Geometry check sheet. Reference: the model listing, model coordinates, mm. A direction names the side the tool comes from. Give positions to 0.01 mm unless a question says otherwise; leave off trailing zeros. Loops run counter-clockwise (first coordinate to the right, second up) from the corner with the lowest first, then second, coordinate; pieces in that order, holes last. Notation, with made-up numbers: (37, 67) -> (67, 67) arc R16 ccw to (67, 85) -> close; hole circle Ø5 at (32, 30.5). An arc over 180 degrees is marked (long way). Write each question's results on one line, items separated by ' | '. Start each with the question number.
1) Draft check along Z on faces 1 (the face through (0, 2, 1)), 2 (the face through (-1, -5.5, 2)), 3 (the face through (0, 0, 4)). Enter one of: pulls with the +Z half, pulls with the -Z half, needs draft (parallel to the pull), parting line crosses it, or undercut.
2) Scan lines: line 1 (Z direction, x = 0, y = -0.75); line 2 (Z direction, x = 0, y = 4.25). Record each from-to range of solid material in increasing order. Write a range as from..to.
3) Sectioned sample at B-B on y = 0. Record the cut outline in (x, z), then the cut area to 3 significant figures.
4) Set-up check for faces 4 (the face through (2, 1.5, -2)), 5 (the face through (2, -1.5, -2)), 6 (the face through (-3.448, 0.021, -2.028)): record each of +Z, -Z, +X, -X, +Y, -Y from which the full face is reachable in a straight line by a thin tool's end or side.
5) Sectioned sample at A-A on x = 0. Record the cut outline in (y, z).
6) Sectioned sample at D-D on z = -3. Record the cut outline in (x, y).
7) Depth check by flat-ended pin: pin 1 (1 mm diameter, centred on x = -3.5, z = -1.5, fed in from +Y); pin 2 (4 mm diameter, centred on x = 2, y = 8, fed in from +Z); pin 3 (1 mm diameter, centred on y = -2.5, z = 0, fed in from -X). Enter the tip coordinate at first touch or a pass-through.
8) Sectioned sample at C-C on x = 3.75. Record the cut outline in (y, z), then the cut area to 3 significant figures.
```python
from build123d import *

# Parameters (mm, degrees)
BOSS_EXTRUDE1_DEPTH = 1.5
SKETCH4_R           = 2.5
BOSS_EXTRUDE3_DEPTH = 4
SKETCH2_R           = 2.5
BOSS_EXTRUDE2_DEPTH = 8
SKETCH3_R           = 1
CUT_EXTRUDE1_DEPTH  = 16
CHAMFER2_SIZE       = 1


with BuildPart() as part:
    # Sketch1 → Boss-Extrude1 (new body, symmetric)
    with BuildSketch(Plane(origin=(0, 0, 0), x_dir=(1, 0, 0), z_dir=(0, 1, 0))):
        Polygon((2.309401077, 4), (-2.309401077, 4), (-4.618802154, 0), (-2.309401077, -4), (2.309401077, -4), (4.618802154, 0), align=None)
    extrude(amount=BOSS_EXTRUDE1_DEPTH, both=True)

    # Sketch4 → Boss-Extrude3 (add)
    with BuildSketch(Plane.XZ.offset(1.5)):
        Circle(SKETCH4_R)
    extrude(amount=BOSS_EXTRUDE3_DEPTH)

    # Sketch2 → Boss-Extrude2 (add)
    with BuildSketch(Plane(origin=(0, 1.5, 0), x_dir=(1, 0, 0), z_dir=(0, 1, 0))):
        Circle(SKETCH2_R)
    extrude(amount=BOSS_EXTRUDE2_DEPTH)

    # Sketch3 → Cut-Extrude1 (cut, through all)
    with BuildSketch(Plane(origin=(0, 9.5, 0), x_dir=(1, 0, 0), z_dir=(0, 1, 0))):
        Circle(SKETCH3_R)
    extrude(amount=-CUT_EXTRUDE1_DEPTH, mode=Mode.SUBTRACT)

    # Chamfer2
    chamfer2_edges = [part.edges().sort_by_distance(p)[0] for p in [
        (-1, -5.5, 0),
        (-1, 9.5, 0),
    ]]
    chamfer(chamfer2_edges, length=CHAMFER2_SIZE)


solid = part.part
```
Result:
1) face 1: undercut | face 2: needs draft | face 3: pulls with the +Z half
2) line 1: -4..-1, 1..4 | line 2: -2.5..-1, 1..2.5
3) outline: (-4.62, 0) -> (-2.31, -4) -> (2.31, -4) -> (4.62, 0) -> (2.31, 4) -> (-2.31, 4) -> close; hole circle Ø2 at (0, 0) | area: 52.3 mm^2
4) face 4: +Y | face 5: -Y | face 6: -Z, -X, +Y, -Y
5) outline: (-5.5, -2.5) -> (-1.5, -2.5) -> (-1.5, -4) -> (1.5, -4) -> (1.5, -2.5) -> (9.5, -2.5) -> (9.5, -2) -> (8.5, -1) -> (-4.5, -1) -> (-5.5, -2) -> close; (-5.5, 2) -> (-4.5, 1) -> (8.5, 1) -> (9.5, 2) -> (9.5, 2.5) -> (1.5, 2.5) -> (1.5, 4) -> (-1.5, 4) -> (-1.5, 2.5) -> (-5.5, 2.5) -> close
6) outline: (-2.89, -1.5) -> (2.89, -1.5) -> (2.89, 1.5) -> (-2.89, 1.5) -> close
7) pin 1: y = 1.5 | pin 2: z = 2.5 | pin 3: x = -2.5
8) outline: (-1.5, -1.5) -> (1.5, -1.5) -> (1.5, 1.5) -> (-1.5, 1.5) -> close | area: 9.03 mm^2
